Geometry: see drawing. Coordinates: mm, zero at the bounding-box minimum. A direction names the side the tool comes from. Coordinates: 2 decimals unless noted, no trailing zeros. Loops run counter-clockwise (first coordinate to the right, second up) from the corner with the lowest first, then second, coordinate; pieces in that order, holes last. Notation, with made-up numbers: (46, 10.25) -> (68, 10.25) arc R24 ccw to (68, 48.25) -> close; hole circle Ø8 at (57.5, -34.75). An arc over 180 degrees is marked (long way). One line per item, written item: value. Start each with the question number.
Item 1: Section query C-C on z = 9. Return loops of the section in (x, y), then the cut area to 3 significant figures.
Item 2: Ray query, probe 1 along X at (y, z) = (91, 14.25). Return the intervals inside material, ascending. Write a range as from..to.
Item 3: Section query B-B on y = 57.5. Return loops of the section in (x, z), then the cut area to 3 significant figures.
Item 4: Section query A-A on x = 16. Return loops of the section in (y, z).
Item 5: Mould query, pull axis X, two halves, no side actions, for the marked faces 1, 2 and 3. Classes: +X half, -X half, draft (parallel to the pull), parting line (faces both ways), or undercut.
Item 6: Contact query for a flat-ended pin moving along its axis: pin 1 Ø10 at (x, z) = (22.5, 17.5) entering from +Y. Output: stop coordinate, or through.
Item 7: Set-up query: the marked faces 4 and 5. Return all of +Z, -Z, +X, -X, +Y, -Y with unobstructed straight access to the full face (end or side cutting, diameter ignored); none if empty.
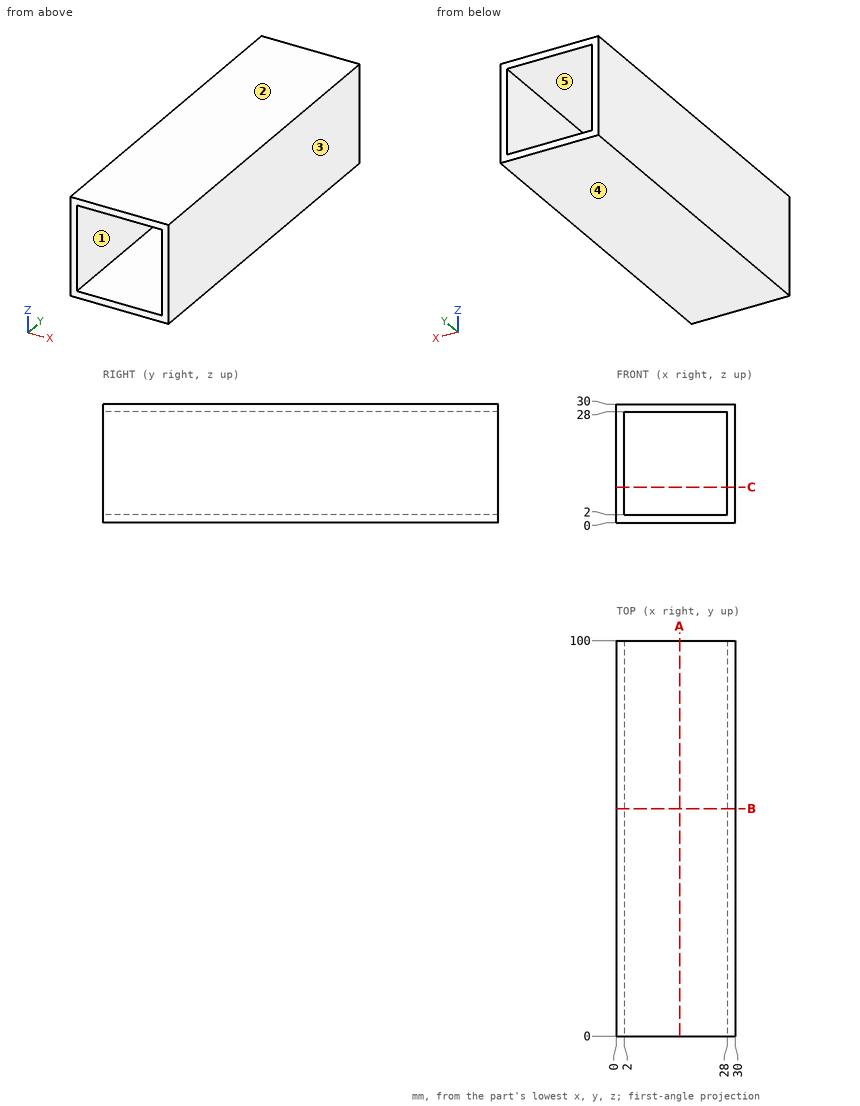
Reply:
1. outline: (0, 0) -> (2, 0) -> (2, 100) -> (0, 100) -> close; (28, 0) -> (30, 0) -> (30, 100) -> (28, 100) -> close
1. area: 400 mm²
2. probe 1: x = 0..2, 28..30
3. outline: (0, 0) -> (30, 0) -> (30, 30) -> (0, 30) -> close; hole (2, 2) -> (28, 2) -> (28, 28) -> (2, 28) -> close
3. area: 224 mm²
4. outline: (0, 0) -> (100, 0) -> (100, 2) -> (0, 2) -> close; (0, 28) -> (100, 28) -> (100, 30) -> (0, 30) -> close
5. face 1: undercut
5. face 2: draft
5. face 3: +X half
6. pin 1: passes through
7. face 4: -Z, +X, -X, +Y, -Y
7. face 5: +Y, -Y
